Geometry check sheet. Reference: the model listing, model coordinates, mm. A direction names the side the tool comes from. Round coordinates to 2 decimals unless told otherwise and drop trailing zeros. Write each loop counter-clockwise with the first axis right and the second up, starting at its lowest first coordinate (ties: lowest second). Pieces come first, ordered by that corner, then holes. Notation, with made-up numbers: (37, 70.25) -> (82, 70.25) arc R19 cw to (82, 100.25) -> close; hole circle Ø4 at (-21, 30). An arc over 180 degrees is marked (long way). Use a Markdown table: item, result.
```python
from build123d import *

# Parameters (mm, degrees)
F0_W      = 419.1
F0_H      = 88.9
F0_R      = 13.096875
F0_R_2    = 11.509375
F0_R_3    = 10.31875
F1_DEPTH  = 12.7
F2_R      = 11.509375
F3_DEPTH  = 12.701
F5_DEPTH  = 12.701
F7_DEPTH  = 12.7010001
F9_DEPTH  = 12.7
F10_R     = 13.096875
F10_R_2   = 11.509375
F10_R_3   = 7.9375
F11_DEPTH = 25.4010001


with BuildPart() as f1:
    # F0 (on Front) → F1 (new body)
    with BuildSketch(Plane.XZ):
        Rectangle(F0_W, F0_H)
        with Locations((-177.8, -12.7)):
            Circle(F0_R, mode=Mode.SUBTRACT)
        with Locations((-12.7, -18.7318846583)):
            Circle(F0_R_2, mode=Mode.SUBTRACT)
        with Locations((19.05, -19.1783625633)):
            Circle(F0_R_2, mode=Mode.SUBTRACT)
        with Locations((50.8, -18.7318846583)):
            Circle(F0_R_2, mode=Mode.SUBTRACT)
        with Locations((82.55, -19.05)):
            Circle(F0_R_2, mode=Mode.SUBTRACT)
        with Locations((133.35, -12.7)):
            Circle(F0_R_3, mode=Mode.SUBTRACT)
        with Locations((184.15, -12.7)):
            Circle(F0_R_3, mode=Mode.SUBTRACT)
    extrude(amount=-F1_DEPTH)

    # F2 (on face) → F3 (cut, through all)
    with BuildSketch(Plane.XZ):
        with Locations((-142.08252, 18.4232164174)):
            Circle(F2_R)
        with Locations((-104.306563735, 14.0248946846)):
            Circle(F2_R)
        with Locations((-71.5190842748, 1.6296281246)):
            Circle(F2_R)
        with Locations((-45.7596568011, -14.1053809535)):
            Circle(F2_R)
    extrude(amount=-F3_DEPTH, mode=Mode.SUBTRACT)

    # F4 (on face) → F5 (cut, through all)
    with BuildSketch(Plane.XZ):
        with BuildLine():
            ThreePointArc((-209.55, -12.7), (-207.0936907923, -0.4549120148), (-200.1048233219, 9.8955162937))
            Line((-200.1048233219, 9.8955162937), (-165.1, 44.45))
            Line((-165.1, 44.45), (-209.55, 44.45))
            Line((-209.55, 44.45), (-209.55, -12.7))
        make_face()
        with BuildLine():
            Line((-209.55, -44.45), (-177.8, -44.45))
            ThreePointArc((-177.8, -44.45), (-200.2506403027, -35.1506403027), (-209.55, -12.7))
            Line((-209.55, -12.7), (-209.55, -44.45))
        make_face()
        with BuildLine():
            ThreePointArc((-146.0861882684, -11.1845312756), (-146.0590483564, -11.9420496313), (-146.05, -12.7))
            ThreePointArc((-146.05, -12.7), (-155.3493596973, -35.1506403027), (-177.8, -44.45))
            Line((-177.8, -44.45), (-38.1, -44.45))
            add(Edge.make_bspline(
                [(-135.731991463, -1.5425124657), (-123.0853934374, -3.2529361125), (-97.8098704079, -7.8915227069), (-55.1757360667, -37.2664877617), (-44.6494842281, -43.1637651569), (-38.1, -44.45)],
                knots=[0, 0, 0, 0, 0.3555356426, 0.7550234425, 1, 1, 1, 1], degree=3))
            ThreePointArc((-135.731991463, -1.5425124657), (-142.8632378904, -4.2650367263), (-146.0861882684, -11.1845312756))
        make_face()
    extrude(amount=-F5_DEPTH, mode=Mode.SUBTRACT)

    # F6 (on face) → F7 (cut, through all)
    with BuildSketch(Plane.XZ):
        with BuildLine():
            Line((209.55, 44.45), (163.5125, 44.45))
            Line((163.5125, 44.45), (202.2463189928, 5.1236707474))
            ThreePointArc((202.2463189928, 5.1236707474), (207.6532604037, -3.0689694011), (209.55, -12.6999998198))
            Line((209.55, -12.6999998198), (209.55, 44.45))
        make_face()
        with BuildLine():
            Line((209.55, -44.45), (209.55, -12.6999998198))
            ThreePointArc((209.55, -12.6999998198), (206.8684506917, -24.0592252451), (199.39, -33.02))
            Line((199.39, -33.02), (184.15, -44.45))
            Line((184.15, -44.45), (209.55, -44.45))
        make_face()
    extrude(amount=-F7_DEPTH, mode=Mode.SUBTRACT)


with BuildPart() as f9:
    # F8 (on Front) → F9 (new body)
    with BuildSketch(Plane.XZ):
        with BuildLine():
            Line((180.975, 31.75), (-180.975, 31.75))
            ThreePointArc((-180.975, 31.75), (-212.725, 0), (-180.975, -31.75))
            Line((-180.975, -31.75), (180.975, -31.75))
            ThreePointArc((180.975, -31.75), (212.725, 0), (180.975, 31.75))
        make_face()
    extrude(amount=F9_DEPTH)

    # F10 (on face) → F11 (cut, through all)
    with BuildSketch(Plane.XZ.offset(12.7)):
        with Locations((-180.975, 0)):
            Circle(F10_R)
        with Locations((-133.35, 0)):
            Circle(F10_R_2)
        with Locations((-107.95, 6.35)):
            Circle(F10_R_2)
        with Locations((-82.55, 7.0877922699)):
            Circle(F10_R_2)
        with Locations((-57.15, 7.0877922699)):
            Circle(F10_R_2)
        with Locations((104.7790011828, 0.7808740327)):
            Circle(F10_R_3)
        with Locations((180.975, 0)):
            Circle(F10_R_3)
    extrude(amount=-F11_DEPTH, mode=Mode.SUBTRACT)


solid = f1.part
```
(1) Access from +Z, -Z, +X, -X, +Y, -Y to the whole of each face (thin tool, end or side, straight path). Record for faces 1 (the face through (-3, 6, 44.45)), 2 (the face through (-142.78, 6.26, -4.19)).
A:
| item | result |
|---|---|
| face 1 | +Z, +X, -X, +Y, -Y |
| face 2 | -Z, +Y, -Y |
(2) Section check B-B on x = 50.8. Record the cut outline in (y, z), plus the area to 3 significant figures.
A:
| item | result |
|---|---|
| outline | (0, -44.45) -> (12.7, -44.45) -> (12.7, -30.24) -> (0, -30.24) -> close; (0, -7.22) -> (12.7, -7.22) -> (12.7, 44.45) -> (0, 44.45) -> close |
| area | 837 mm2 |
(3) Gauge pin test, flat ends, axial feed: pin 1 Ø6 at (y, z) = (1.5, -20) entering from -X; pin 2 Ø1.5 at (x, y) = (-164, 4.5) entering from -Z; pin 3 Ø2 at (y, z) = (7, 0.5) entering from -X. Record the tip position at first contact, or that the pin passes through.
A:
| item | result |
|---|---|
| pin 1 | stops at x = -209.26 |
| pin 2 | stops at z = -41.64 |
| pin 3 | stops at x = -207.11 |
(4) Release check for a two-part mould opening along X. For faces 3 (the face through (-60.541, 6.261, 5.087)), 4 (the face through (143.19, 6.26, -9.6)), 5 (the face through (-182.85, 6.26, 26.93)), 6 (the face through (71, 6, -44.45)) record: +X half, -X half, draft (parallel to the pull), parting line (faces both ways), or undercut.
A:
| item | result |
|---|---|
| face 3 | undercut |
| face 4 | undercut |
| face 5 | -X half |
| face 6 | draft |
(5) Section check C-C on y = 9. State how many separate pieces and enclosed holes the cut face has, plus the area to 3 significant figures.
A:
| item | result |
|---|---|
| separate pieces | 1 |
| enclosed holes | 11 |
| area | 27,100 mm2 |
(6) Section check A-A on x = 133.35. Record the cut outline in (y, z), plus the area to 3 significant figures.
A:
| item | result |
|---|---|
| outline | (0, -44.45) -> (12.7, -44.45) -> (12.7, -23.02) -> (0, -23.02) -> close; (0, -2.38) -> (12.7, -2.38) -> (12.7, 44.45) -> (0, 44.45) -> close |
| area | 867 mm2 |
(7) Thickness scan on line 1 (Z direction, x = 19.05, y = 7.75); line 2 (X direction, y = 3.5, z = 21.5); line 3 (X direction, y = 5.5, z = -33). Record the ranges inside material, lowest first.
A:
| item | result |
|---|---|
| line 1 | z = -44.45 to -30.69, -7.67 to 44.45 |
| line 2 | x = -188.35 to -153.17, -130.99 to -113.06, -95.56 to 186.12 |
| line 3 | x = -202.21 to -153.39, -60.96 to 199.42 |
